```python
from build123d import *

# Parameters (mm, degrees)
SKETCH_1_R               = 16
SKETCH_1_R_2             = 4
EXTRUDE_1_DEPTH          = 10
SKETCH_2_R               = 2.5
CUT_EXTRUDE_1_DEPTH      = 20
PATTERN_CIRCULAR_1_COUNT = 8
SKETCH_3_R               = 7
CUT_EXTRUDE_2_DEPTH      = 5
SKETCH_4_R               = 6
CUT_EXTRUDE_3_DEPTH      = 1
EXTRUDE_START            = 20
SKETCH_5_R               = 16
SKETCH_5_R_2             = 14
EXTRUDE_2_DEPTH          = 20


with BuildPart() as part:
    # 스케치1 → 보스-돌출1 (new body)
    with BuildSketch(Plane.XY):
        Circle(SKETCH_1_R)
        Circle(SKETCH_1_R_2, mode=Mode.SUBTRACT)
    extrude(amount=EXTRUDE_1_DEPTH)

    # 스케치2 → 컷-돌출1 (cut)
    with BuildSketch(Plane.XY):
        with Locations((0, 11)):
            Circle(SKETCH_2_R)
    cut_extrude_1 = extrude(amount=CUT_EXTRUDE_1_DEPTH, mode=Mode.SUBTRACT)

    # 원형 패턴1: 컷-돌출1 ×8 about axis
    pattern_circular_1_axis = Axis((0, 0, 0), (0, 0, 1))
    for i in range(1, PATTERN_CIRCULAR_1_COUNT):
        add(cut_extrude_1.rotate(pattern_circular_1_axis, i * 360 / PATTERN_CIRCULAR_1_COUNT), mode=Mode.SUBTRACT)

    # 스케치3 → 컷-돌출2 (cut)
    with BuildSketch(Plane.XY.offset(10)):
        Circle(SKETCH_3_R)
    extrude(amount=-CUT_EXTRUDE_2_DEPTH, mode=Mode.SUBTRACT)

    # 스케치4 → 컷-돌출3 (cut)
    with BuildSketch(Plane(origin=(0, 0, 0), x_dir=(-1, 0, 0), z_dir=(0, 0, -1))):
        Circle(SKETCH_4_R)
    extrude(amount=-CUT_EXTRUDE_3_DEPTH, mode=Mode.SUBTRACT)

    # 스케치5 → 보스-돌출2 (add)
    with BuildSketch(Plane(origin=(0, 0, 0), x_dir=(-1, 0, 0), z_dir=(0, 0, -1)).offset(EXTRUDE_START)):
        Circle(SKETCH_5_R)
        Circle(SKETCH_5_R_2, mode=Mode.SUBTRACT)
    extrude(amount=-EXTRUDE_2_DEPTH)

    # 스케치6 → 회전1 (revolve)
    with BuildSketch(Plane(origin=(0, 0, 0), x_dir=(0, 0, -1), z_dir=(1, 0, 0)), mode=Mode.PRIVATE) as revolve_1_sk:
        Polygon((20, 14), (20, 6.1), (9.414853381, 6.1), (0, 13.5), (0, 14), align=None)
    revolve(revolve_1_sk.sketch.rotate(Axis((0, 0, 0), (0, 0, -1)), 270), axis=Axis((0, 0, 0), (0, 0, -1)))


solid = part.part
```
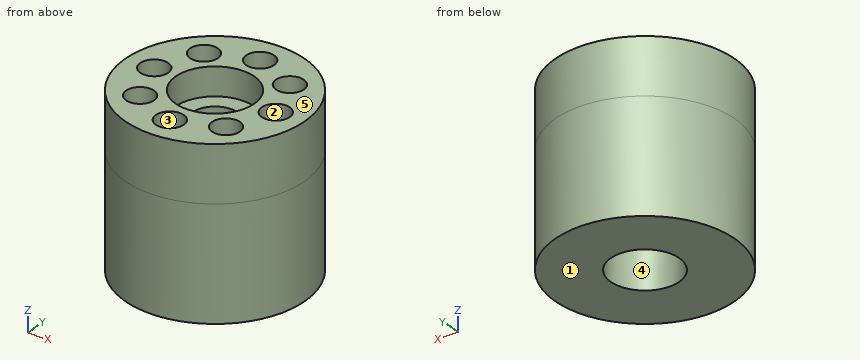
Geometry: final body of the model. Coordinates: model frame, mm. Face numbers are marked on the shaded views. A direction names the side the tool comes from. Give positions to 0.01 mm unless a question says otherwise; leave off trailing zeros. Order: outer loops, then holes, each group sorted by start corner. A loop starts at its lowest first (then second) coordinate and runs counter-clockwise, first axis right, second up. Notation, with made-up numbers: (-2.5, 24) -> (1.5, 24) arc R13 ccw to (1.5, 39) -> close; hole circle Ø10 at (-37, 0.25). An arc over 180 degrees is marked (long way). Write each question's results on one line, items separated by ' | '. Start each with the question number.
1) Draft query along Y for the marked faces 1 and 2. Return one class per face: pulls with the +Y half, pulls with the -Y half, needs draft (parallel to the pull), parting line crosses it, or undercut.
2) Section A-A (z = 6). Count the separate pieces of the cut face and the enclosed holes in it, then the cut area to 3 significant figures.
3) First-contact query: pin 1 (4 mm diameter, centred on y = 7, z = -4.5, fed in from +X); pin 2 (4.5 mm diameter, centred on x = -7.78, y = -7.78, fed in from +Z); pin 3 (3 mm diameter, centred on y = -6, z = 4, fed in from +X). Flat tips, straight axial feed; report the tip coordinate or a pass-through.
4) Line query: line 1 (Y direction, x = 0, z = 2.9); line 2 (X direction, y = 10, z = 0.25); line 3 (X direction, y = -1.5, z = 6). Output: solid intervals per line, ascending. Write a range as from..to.
5) Set-up query: the marked faces 3, 4 and 5. Return all of +Z, -Z, +X, -X, +Y, -Y with unobstructed straight access to the full face (end or side cutting, diameter ignored); none if empty.
6) Section D-D (z = -2.5). Return loops of the section in (x, y).
Calculated:
1) face 1: needs draft | face 2: undercut
2) separate pieces: 1 | enclosed holes: 9 | area: 493 mm2
3) pin 1: x = 15.2 | pin 2: z = -0.31 | pin 3: x = 15.35
4) line 1: -16..-13.5, -8.5..-4, 4..8.5, 13.5..16 | line 2: -12.49..-8.92, -6.63..-2.29, 2.29..6.63, 8.92..12.49 | line 3: -15.93..-13, -9..-6.84, 6.84..9, 13..15.93
5) face 3: +Z | face 4: -Z | face 5: +Z, +X, -X, +Y, -Y
6) outline: circle Ø32 at (0, 0); hole circle Ø23.07 at (0, 0)
